Design review of the part built by this model. Coordinates are the model's own, in mm. A direction names the side the tool comes from. Give positions to 0.01 mm unless a question says otherwise; leave off trailing zeros. Order: outer loops, then holes, each group sorted by start corner. A loop starts at its lowest first (then second) coordinate and runs counter-clockwise, first axis right, second up. Notation, with made-up numbers: (79.5, 71) -> (109.5, 71) arc R17 ccw to (109.5, 99) -> close; hole circle Ø5 at (-19.5, 24.5). An arc over 180 degrees is marked (long way). One line per item, written item: value.
from build123d import *

# Parameters (mm, degrees)
SKETCH1_W          = 52.8624
SKETCH1_H          = 22.352
BASE_FLANGE1_DEPTH = 3.175
CUT_EXTRUDE1_DEPTH = 3.175
FILLET1_R          = 6.35


# Sheet-metal steps are written as plain solids
with BuildPart() as part:
    # Sketch1 → Base-Flange1 (new body)
    with BuildSketch(Plane.XY):
        with Locations((26.4312, 11.176)):
            Rectangle(SKETCH1_W, SKETCH1_H)
    extrude(amount=-BASE_FLANGE1_DEPTH)

    # Sketch6 → Cut-Extrude1 (cut)
    with BuildSketch(Plane.XY):
        with BuildLine():
            Line((7.325, 13.926), (12.325, 13.926))
            ThreePointArc((12.325, 13.926), (15.075, 11.176), (12.325, 8.426))
            Line((12.325, 8.426), (7.325, 8.426))
            ThreePointArc((7.325, 8.426), (4.575, 11.176), (7.325, 13.926))
        make_face()
        with BuildLine():
            Line((42.9437, 6.8072), (43.7311, 6.8072))
            ThreePointArc((43.7311, 6.8072), (48.0999, 11.176), (43.7311, 15.5448))
            Line((43.7311, 15.5448), (42.9437, 15.5448))
            ThreePointArc((42.9437, 15.5448), (38.5749, 11.176), (42.9437, 6.8072))
        make_face()
    extrude(amount=-CUT_EXTRUDE1_DEPTH, mode=Mode.SUBTRACT)

    # Fillet1
    fillet1_edges = [part.edges().sort_by_distance(p)[0] for p in [
        (0, 22.352, -1.5875),
        (52.8624, 22.352, -1.5875),
        (52.8624, 0, -1.5875),
        (0, 0, -1.5875),
    ]]
    fillet(fillet1_edges, radius=FILLET1_R)


solid = part.part
Item 1: Add section C-C on z = -1.2. Give the boundary of the cut face in (x, y) (3 decimals).
Returned:
outline: (0, 6.35) arc R6.35 ccw to (6.35, 0) -> (46.512, 0) arc R6.35 ccw to (52.862, 6.35) -> (52.862, 16.002) arc R6.35 ccw to (46.512, 22.352) -> (6.35, 22.352) arc R6.35 ccw to (0, 16.002) -> close; hole (7.325, 8.426) -> (12.325, 8.426) arc R2.75 ccw to (12.325, 13.926) -> (7.325, 13.926) arc R2.75 ccw to start; hole (42.944, 6.807) -> (43.731, 6.807) arc R4.369 ccw to (43.731, 15.545) -> (42.944, 15.545) arc R4.369 ccw to start
Item 2: Machinability: for faces 5 (the flat face through (10, 8.426, -2)), 6 (the cylindrical face through (1.81, 20.44, -1.61)), which of the approach directions +Z, -Z, +X, -X, +Y, -Y give a long, thin tool a straight path to every point of the face, cutting with its end or side? Answer none if there is none.
Returned:
face 5: +Z, -Z
face 6: +Z, -Z, -X, +Y
Item 3: Add section D-D on y = 14.75. Give the boundary of the cut face in (x, z) (3 decimals).
Returned:
outline: (0, -3.175) -> (40.431, -3.175) -> (40.431, 0) -> (0, 0) -> close; (46.244, -3.175) -> (52.862, -3.175) -> (52.862, 0) -> (46.244, 0) -> close
Item 4: To check wall thickness, follow line 1 along X through (y, z) = (6, -1.1); line 2 along Y through (x, z) = (39, -0.85); line 3 along X through (y, z) = (12.75, -1.8). State the ranges of each line that lie inside material, in increasing order. Write a range as from..to.
Returned:
line 1: 0.01..52.85
line 2: 0..9.3, 13.06..22.35
line 3: 0..5.07, 14.58..38.87, 47.81..52.86
Item 5: Add section A-A on x = 11.5. Give the boundary of the cut face in (y, z) (3 decimals), plus the area to 3 significant figures.
Returned:
outline: (0, -3.175) -> (8.426, -3.175) -> (8.426, 0) -> (0, 0) -> close; (13.926, -3.175) -> (22.352, -3.175) -> (22.352, 0) -> (13.926, 0) -> close
area: 53.5 mm²
Item 6: Draft analysis for pull direction Y (two halves, no side actions). For faces 1 (the flat face through (10, 13.926, -2)), 2 (the cylindrical face through (4.576, 11.116, -1.565)), 3 (the flat face through (26, 22.352, -2)), 4 (the flat face through (52.862, 11, -2)), state which applies: pulls with the +Y half, pulls with the -Y half, needs draft (parallel to the pull), parting line crosses it, or undercut.
Returned:
face 1: undercut
face 2: undercut
face 3: pulls with the +Y half
face 4: needs draft
Item 7: Add section B-B on y = 11. Give the boundary of the cut face in (x, z) (3 decimals), plus the area to 3 significant figures.
Returned:
outline: (0, -3.175) -> (4.581, -3.175) -> (4.581, 0) -> (0, 0) -> close; (15.069, -3.175) -> (38.578, -3.175) -> (38.578, 0) -> (15.069, 0) -> close; (48.096, -3.175) -> (52.862, -3.175) -> (52.862, 0) -> (48.096, 0) -> close
area: 104 mm²
